Could you check a few things on this drawing? It's one solid part, dimensions in mm from its lowest x, y, z. A direction names the side the tool comes from. Round coordinates to 2 decimals unless told otherwise and drop trailing zeros. Write each loop counter-clockwise with the first axis right and the second up, starting at its lowest first coordinate (ties: lowest second). Pieces come first, ordered by that corner, then holes. Notation, with made-up numbers: (3.25, 4.5) -> (32.25, 4.5) arc R15 cw to (32.25, 28.5) -> close; hole circle Ø9 at (14, 43). An arc over 180 degrees is marked (long way). Answer in a Markdown table with one row per item. Add a question column.
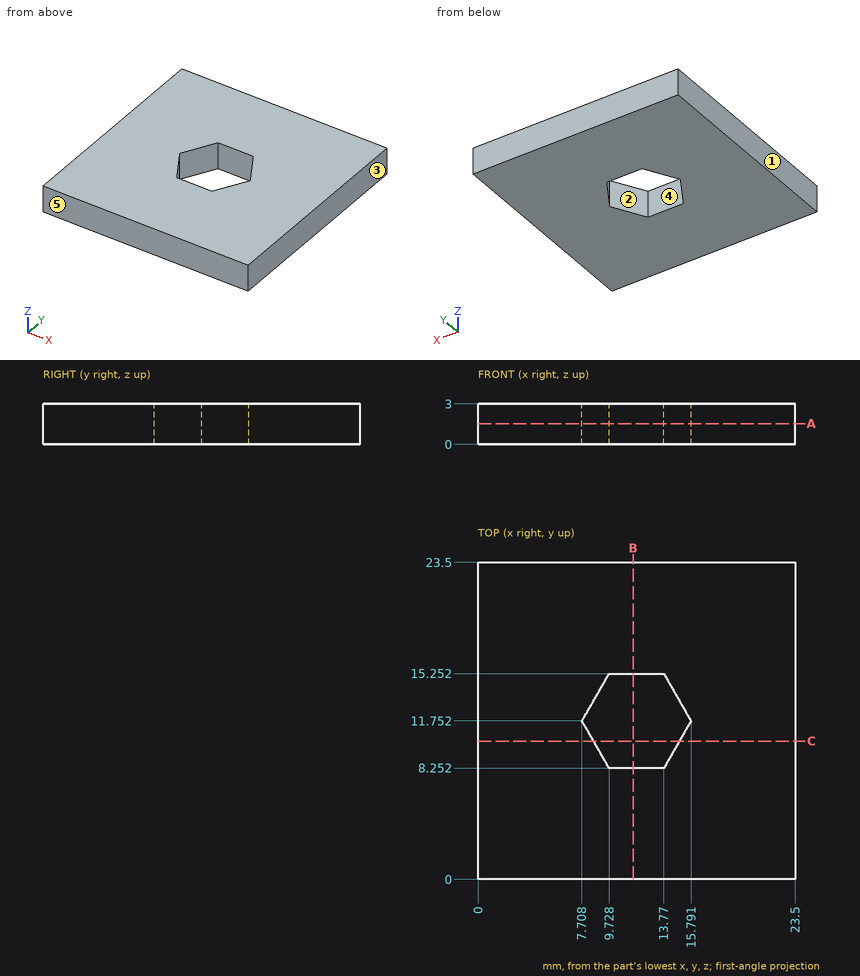
Item 1: If we mould it in two halves opening along Y, with no side actions, what happens to the marked faces 3, 4 and 5? For each: pulls with the +Y half, pulls with the -Y half, needs draft (parallel to the pull), parting line crosses it, or undercut.
Item 2: For P1, Ø1, axis at y = 15.5, z = 1, coming from the -X side, with a flat end and sliding along its axis, tell me the tip position at first contact or that it passes through.
Item 3: If we section it at C-C on y = 10.25: Please give me the cut outline in (x, z) (1 decimal).
Item 4: On a 3-axis mill with a long thin cutter (end or side, diameter ignored), from which of +Z, -Z, +X, -X, +Y, -Y can I reach the whole of each face in a straight line? I mean the marked faces 1 and 2. Say none if no direction works.
Item 5: If we section it at B-B on x = 11.5: Please give me the cut outline in (y, z), then the cut area to 3 significant figures.
Item 6: If we section it at A-A on z = 1.55: Please give me the cut outline in (x, y), then the cut area to 3 significant figures.
Item 7: I need wall thicknesses on line 1 along Y through (x, z) = (11.75, 2.85); line 2 along X through (y, z) = (9.5, 1.7); line 3 along Y through (x, z) = (9.25, 2.6) (1 decimal). Which ranges of each line are inside material? Lowest first, please. Write a range as from..to.
Results list:
| question | item | result |
|---|---|---|
| 1 | face 3 | needs draft |
| 1 | face 4 | undercut |
| 1 | face 5 | pulls with the -Y half |
| 2 | P1 | x = 0 |
| 3 | outline | (0, 0) -> (8.6, 0) -> (8.6, 3) -> (0, 3) -> close; (14.9, 0) -> (23.5, 0) -> (23.5, 3) -> (14.9, 3) -> close |
| 4 | face 1 | +Z, -Z, -X, +Y, -Y |
| 4 | face 2 | +Z, -Z |
| 5 | outline | (0, 0) -> (8.25, 0) -> (8.25, 3) -> (0, 3) -> close; (15.25, 0) -> (23.5, 0) -> (23.5, 3) -> (15.25, 3) -> close |
| 5 | area | 49.5 mm² |
| 6 | outline | (0, 0) -> (23.5, 0) -> (23.5, 23.5) -> (0, 23.5) -> close; hole (7.71, 11.75) -> (9.73, 8.25) -> (13.77, 8.25) -> (15.79, 11.75) -> (13.77, 15.25) -> (9.73, 15.25) -> close |
| 6 | area | 510 mm² |
| 7 | line 1 | 0..8.25, 15.25..23.5 |
| 7 | line 2 | 0..9.01, 14.49..23.5 |
| 7 | line 3 | 0..9.1, 14.4..23.5 |
